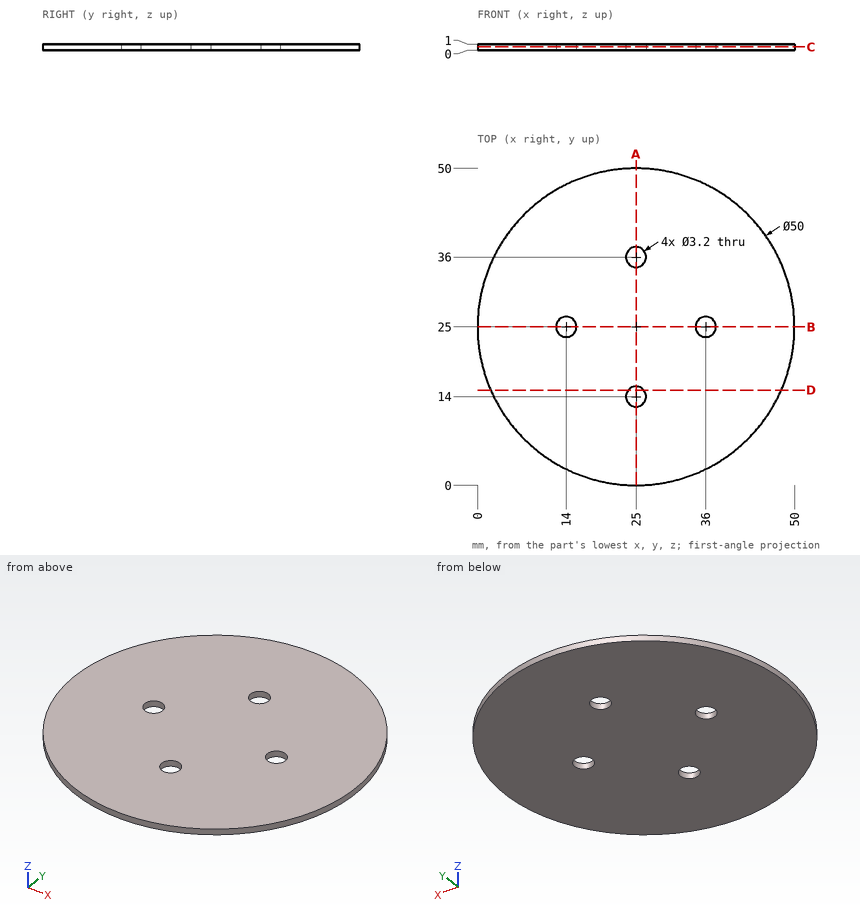
Job drawing, mm, ordinate dimensions from the low corner. One solid piece. Give positions to 0.01 mm unless a question says otherwise; leave off trailing zeros. Loops run counter-clockwise (first coordinate to the right, second up) from the corner with the lowest first, then second, coordinate; pieces in that order, holes last. Notation, with made-up numbers: (18, 67) -> (65, 67) arc R11 cw to (65, 85) -> close; hole circle Ø3 at (81, 4.25). An arc over 180 degrees is marked (long way). Write each question's results on one line, items separated by ' | '.
(1) Cut at C-C on z = 0.55. List the corners of the cut face in (x, y).
Geometry results:
outline: circle Ø50 at (25, 25); hole circle Ø3.2 at (14, 25); hole circle Ø3.2 at (25, 14); hole circle Ø3.2 at (25, 36); hole circle Ø3.2 at (36, 25)
(2) Cut at A-A on x = 25. List the corners of the cut face in (y, z).
Geometry results:
outline: (0, 0) -> (12.4, 0) -> (12.4, 1) -> (0, 1) -> close; (15.6, 0) -> (34.4, 0) -> (34.4, 1) -> (15.6, 1) -> close; (37.6, 0) -> (50, 0) -> (50, 1) -> (37.6, 1) -> close
(3) Cut at D-D on y = 15. List the corners of the cut face in (x, z), and give its area (3 significant figures).
Geometry results:
outline: (2.09, 0) -> (23.75, 0) -> (23.75, 1) -> (2.09, 1) -> close; (26.25, 0) -> (47.91, 0) -> (47.91, 1) -> (26.25, 1) -> close | area: 43.3 mm²
(4) Probe line 1 along X through (y, z) = (25, 0.35); line 2 along Y through (x, z) = (25.5, 0.6) (3 decimals). List the from-to ranges inside material, lowest first.
Geometry results:
line 1: x = 0 to 12.4, 15.6 to 34.4, 37.6 to 50 | line 2: y = 0.005 to 12.48, 15.52 to 34.48, 37.52 to 49.995
